Model file for the job. Use its own axes, mm. A direction names the side the tool comes from. Round coordinates to 2 decimals unless told otherwise and drop trailing zeros. Loops run counter-clockwise (first coordinate to the right, second up) from the corner with the lowest first, then second, coordinate; pieces in that order, holes last. Notation, with made-up numbers: M 28.5,5.5 L 83.5,5.5 A21 ccw 83.5,30.5 Z; hole C -30,-11.5 d10. An arc over 180 degrees is marked long. Use a Markdown table: item, result. Add a question column.
Item 1: Saw through at C-C on z = -7. Write the cut outline in (x, y), then the cut area to 3 significant figures.
Item 2: Pin check, flat tips, straight feed: P1, Ø1, axis at y = 40.5, z = -19, coming from the -X side; P2, Ø5, axis at y = 42.5, z = -25, coming from the +X side; P3, Ø6, axis at y = 43, z = -11, coming from the -X side; P4, Ø3, axis at x = -7.5, y = 35, coming from the -Z side. Stop position of each tip, or through.
Item 3: Tool access for faces 4 (the flat face through (-12.6, 4, -12.6)), 5 (the flat face through (0, 1, -23)): list every direction of +Z, -Z, +X, -X, +Y, -Y with a clear straight run to the whole face (end or side of a thin tool).
Item 4: Two-plate mould, pull along Z, no slides. Class faces 1 (the flat face through (-22, 1, 0)), 2 (the cylindrical face through (-44.43, 1.48, -44.4)), 3 (the cylindrical face through (-21.84, 26.62, -12.52)): +Z half, -Z half, draft (parallel to the pull), parting line (faces both ways), or undercut.
Item 5: Saw through at A-A on y = 17.5. Write the cut outline in (x, z), then the cut area to 3 significant figures.
Item 6: Wall check: L1, parallel to X at y = 22.5, z = -22.5; L2, parallel to Z at x = -19.5, y = 47. Give the ranges that are in metal, low to high. Write a range as from..to.
Item 7: Saw through at D-D on x = -41. Write the cut outline in (y, z).
Autodesk Inventor part; units mm, degrees
ref_plane "YZ Plane" through (0, 0, 0) normal (1, 0, 0) x (0, 1, 0)
ref_plane "XZ Plane" through (0, 0, 0) normal (0, 1, 0) x (-1, 0, 0)
ref_plane "XY Plane" through (0, 0, 0) normal (0, 0, 1) x (1, 0, 0)
sketch "底面" plane through (0, 0, 0) normal (0, 1, 0) x (-1, 0, 0)
  line L0 (2, 0) -> (43, 0)
  line L1 (45, -2) -> (45, -43)
  line L2 (43, -45) -> (2, -45)
  line L3 (0, -43) -> (0, -2)
  arc A0 (45, -2) -> (43, 0) centre (43, -2) ccw
  arc A1 (43, -45) -> (45, -43) centre (43, -43) ccw
  arc A2 (0, -43) -> (2, -45) centre (2, -43) ccw
  arc A3 (2, 0) -> (0, -2) centre (2, -2) ccw
  circle A4 centre (22.5, -22.5) radius 10
  point P0 (0, 0)
  point P1 (45, -45)
  point P2 (45, 0)
  point P3 (0, -45)
  point P4 (45, -22.5)
  point P5 (22.5, 0)
  dimension "d0" = 45
  dimension "d1" = 45
  dimension "d2" = 2
  dimension "d8" = 20
extrude "底" add sketch "底面" along normal blind 4
sketch "スケッチ2" plane through (0, 4, 0) normal (0, 1, 0) x (1, 0, 0)
  circle A0 centre (-22.5, 22.5) radius 12.5
  line L0 (-43, 0) -> (-2, 0)
  line L1 (-45, 43) -> (-45, 2)
  circle A1 centre (-22.5, 22.5) radius 10
  point P0 (0, 0)
  point P1 (-22.5, 0)
  point P2 (-45, 22.5)
  dimension "d5" = 25
extrude "棒" add sketch "スケッチ2" along normal blind 50
fillet "フィレット1" radius 1 2 edges at (-35, 4, -22.5) (-35, 54, -22.5)
fillet "フィレット2" radius 1 8 edges at (-0.5858, 4, -0.5858) (0, 4, -22.5) (-0.5858, 4, -44.4142) (-22.5, 4, -45) (-44.4142, 4, -44.4142) (-45, 4, -22.5) (-44.4142, 4, -0.5858) (-22.5, 4, 0)
properties part number "pole-2_3D プリント"
Entries:
| question | item | result |
|---|---|---|
| 1 | outline | M -45,0 L 0,0 L 0,3 A1 ccw -1,4 L -44,4 A1 ccw -45,3 Z |
| 1 | area | 180 mm2 |
| 2 | P1 | x = -34.63 |
| 2 | P2 | x = -10 |
| 2 | P3 | x = -31.67 |
| 2 | P4 | through |
| 3 | face 4 | +Y |
| 3 | face 5 | +Z, -Z, +X, +Y, -Y |
| 4 | face 1 | +Z half |
| 4 | face 2 | -Z half |
| 4 | face 3 | undercut |
| 5 | outline | C -22.5,-22.5 d25; hole C -22.5,-22.5 d20 |
| 5 | area | 177 mm2 |
| 6 | L1 | -35..-32.5, -12.5..-10 |
| 6 | L2 | -34.63..-32.04, -12.96..-10.37 |
| 7 | outline | M 0,-45 L 3,-45 A1 ccw 4,-44 L 4,-1 A1 ccw 3,0 L 0,0 Z |
